from build123d import *

# Parameters (mm, degrees)
F0_W      = 6
F0_H      = 2
F1_DEPTH  = 6
F2_W      = 6
F2_H      = 6
F3_DEPTH  = 10
F4_W      = 24
F4_H      = 12
F5_DEPTH  = 6
F7_DEPTH  = 12.001
F8_W      = 6.1598163333
F8_H      = 6
F9_DEPTH  = 15
F10_W     = 6
F10_H     = 2.5150536597
F11_DEPTH = 4
F12_W     = 24.6021291241
F12_H     = 7.3056968898
F13_DEPTH = 6
F14_W     = 5.5018218607
F14_H     = 5.5230222642
F15_DEPTH = 24.6031291241
F16_R     = 1.5
F17_DEPTH = 1
F18_W     = 2.4501711503
F18_H     = 3.5
F18_W_2   = 2.5247114152
F18_W_3   = 2.5247123465
F19_DEPTH = 5


with BuildPart() as f1:
    # F0 (on Top) → F1 (new body)
    with BuildSketch(Plane.XY):
        with Locations((-32.0476180848, -1)):
            Rectangle(F0_W, F0_H)
    extrude(amount=F1_DEPTH)

    # F2 (on face) → F3 (join)
    with BuildSketch(Plane.YZ.offset(-29.0476180848)):
        with Locations((-1.0433437443, 3)):
            Rectangle(F2_W, F2_H)
    extrude(amount=F3_DEPTH)

    # F4 (on face) → F5 (join)
    with BuildSketch(Plane.YZ.offset(-19.0476180848)):
        with Locations((-1.0433437443, 3)):
            Rectangle(F4_W, F4_H)
    extrude(amount=F5_DEPTH)

    # F6 (on face) → F7 (cut, through all)
    with BuildSketch(Plane.XY.offset(9)):
        with BuildLine():
            Line((-13.0476180848, -11.1071496376), (-13.0476180848, -7.6019221608))
            ThreePointArc((-13.0476180848, -7.6019221608), (-16.5476180848, -9.3545358992), (-13.0476180848, -11.1071496376))
        make_face()
        with BuildLine():
            ThreePointArc((-13.0476180848, 0.4656811595), (-16.5476180848, -1.0765416363), (-13.0476180848, -2.618764432))
            Line((-13.0476180848, -2.618764432), (-13.0476180848, 0.4656811595))
        make_face()
        with BuildLine():
            ThreePointArc((-13.0476180848, 9.0525666852), (-16.5476180848, 7.234418936), (-13.0476180848, 5.4162711868))
            Line((-13.0476180848, 5.4162711868), (-13.0476180848, 9.0525666852))
        make_face()
    extrude(amount=-F7_DEPTH, mode=Mode.SUBTRACT)

    # F8 (on face) → F9 (join)
    with BuildSketch(Plane.XY.offset(6)):
        with Locations((-25.9677099181, -1.0433437443)):
            Rectangle(F8_W, F8_H)
    extrude(amount=F9_DEPTH)

    # F10 (on face) → F11 (join)
    with BuildSketch(Plane.YZ.offset(-22.8878017515)):
        with Locations((-1.0433437443, 19.7424731702)):
            Rectangle(F10_W, F10_H)
    extrude(amount=F11_DEPTH)

    # F12 (on face) → F13 (join)
    with BuildSketch(Plane.YZ.offset(-18.8878017515)):
        with Locations((-0.8769654669, 17.3471515551)):
            Rectangle(F12_W, F12_H)
    extrude(amount=F13_DEPTH)

    # F14 (on face) → F15 (cut, through all)
    with BuildSketch(Plane(origin=(0, 11.4240990952, 0), x_dir=(-1, 0, 0), z_dir=(0, 1, 0))):
        with Locations((15.6387126818, 17.3303969204)):
            Rectangle(F14_W, F14_H)
    extrude(amount=-F15_DEPTH, mode=Mode.SUBTRACT)

    # F16 (on face) → F17 (cut)
    with BuildSketch(Plane.XY.offset(14.5688857883)):
        with Locations((-13.8878017515, -9.5042175321)):
            Circle(F16_R)
        with Locations((-13.8878017515, -1.0522056698)):
            Circle(F16_R)
        with Locations((-13.8878017515, 7.322568293)):
            Circle(F16_R)
    extrude(amount=-F17_DEPTH, mode=Mode.SUBTRACT)

    # F18 (on face) → F19 (join)
    with BuildSketch(Plane(origin=(0, 0, 20.0919080526), x_dir=(1, 0, 0), z_dir=(0, 0, -1))):
        with Locations((-14.1128873266, -7.338691324)):
            Rectangle(F18_W, F18_H)
        with Locations((-14.1501574591, 1.0843175156)):
            Rectangle(F18_W_2, F18_H)
        with Locations((-14.1501579247, 9.5073256567)):
            Rectangle(F18_W_3, F18_H)
    extrude(amount=F19_DEPTH)


solid = f1.part
The listing builds one solid part. Answer for the finished solid, in the listing's coordinates (mm). A direction names the side the tool comes from. Round coordinates to 2 decimals unless told otherwise and drop trailing zeros. Write each loop counter-clockwise with the first axis right and the second up, starting at its lowest first coordinate (ties: lowest second). Pieces come first, ordered by that corner, then holes. Notation, with made-up numbers: (-26.5, 77.25) - (27.5, 77.25) arc R25 ccw to (27.5, 104.25) - close; hole circle Ø8 at (54.5, 40). An arc over 180 degrees is marked (long way). Use a Markdown table: item, result. Add a question column.
1. The part is cut by section A-A (y = -6.75). Write down the section's boundary in (x, z), and give its area (3 significant figures).
2. Consider line 1 (Y direction, x = -14.5, z = 6.5); line 2 (Z direction, x = -16, y = 2.5); line 3 (X direction, y = 1, z = 15.5). Determine where each line is inside the solid, lowest interval first.
3. A tool of negligible diameter and unlimited length cuts with its end or side. For faces 5 (the face through (-15.413, -9, 18)), 6 (the face through (-15.387, 7.371, 14.138)), 7 (the face through (-32, -1, 6)), from which of +Z, -Z, +X, -X, +Y, -Y can it reach the whole face along a straight path? Write none if from no direction.
4. The part is cut by section B-B (z = 5.5). Write down the section's boundary in (x, y), and give its area (3 significant figures).
5. The part is cut by section D-D (x = -28.5). Write down the section's boundary in (y, z).
6. For a pull along Z with two mould halves and no side action, classify faces 1 (the face through (-21, -1, 6)), 2 (the face through (-25, -1, 0)), 3 (the face through (-12.888, 10, 14)), 4 (the face through (-19, -1, 21)) as +Z half, -Z half, draft (parallel to the pull), parting line (faces both ways), or undercut.
7. The part is cut by section C-C (x = -15.75). Write down the section's boundary in (y, z).
8. Flat-ended cylindrical pins translate along their axes: P1, Ø5, axis at y = 0, z = 10, coming from the -X side; P2, Ø2, axis at x = -14.5, y = -2, coming from the -Z side; P3, Ø2, axis at x = -32.5, y = -1, coming from the +Z side; P4, Ø12, axis at y = 3, z = 4.5, coming from the -X side. Find the tip coordinate at first contact, or state that the pin passes through.
Reported:
| question | item | result |
|---|---|---|
| 1 | outline | (-19.05, -3) - (-13.05, -3) - (-13.05, 9) - (-19.05, 9) - close; (-18.89, 13.69) - (-12.89, 13.69) - (-12.89, 14.57) - (-18.39, 14.57) - (-18.39, 20.09) - (-12.89, 20.09) - (-12.89, 21) - (-18.89, 21) - close |
| 1 | area | 85.4 mm^2 |
| 2 | line 1 | -13.04 to -11.54, -7.17 to -3.17, 1.01 to 5.02, 9.45 to 10.96 |
| 2 | line 2 | -3 to 9, 13.69 to 14.57, 20.09 to 21 |
| 2 | line 3 | -29.05 to -22.89, -18.89 to -18.39 |
| 3 | face 5 | +Y, -Y |
| 3 | face 6 | -Z |
| 3 | face 7 | +Z, -X, +Y, -Y |
| 4 | outline | (-35.05, -2) - (-29.05, -2) - (-29.05, -4.04) - (-19.05, -4.04) - (-19.05, -13.04) - (-13.05, -13.04) - (-13.05, -11.11) arc R2.19 cw (long way) to (-13.05, -7.6) - (-13.05, -2.62) arc R2.09 cw (long way) to (-13.05, 0.47) - (-13.05, 5.42) arc R2.22 cw (long way) to (-13.05, 9.05) - (-13.05, 10.96) - (-19.05, 10.96) - (-19.05, 1.96) - (-29.05, 1.96) - (-29.05, 0) - (-35.05, 0) - close |
| 4 | area | 178 mm^2 |
| 5 | outline | (-4.04, 0) - (1.96, 0) - (1.96, 21) - (-4.04, 21) - close |
| 6 | face 1 | undercut |
| 6 | face 2 | -Z half |
| 6 | face 3 | draft |
| 6 | face 4 | +Z half |
| 7 | outline | (-13.18, 13.69) - (11.42, 13.69) - (11.42, 14.57) - (-13.18, 14.57) - close; (-13.18, 20.09) - (11.42, 20.09) - (11.42, 21) - (-13.18, 21) - close; (-13.04, -3) - (-11.04, -3) - (-11.04, 9) - (-13.04, 9) - close; (-7.66, -3) - (-2.72, -3) - (-2.72, 9) - (-7.66, 9) - close; (0.57, -3) - (5.53, -3) - (5.53, 9) - (0.57, 9) - close; (8.94, -3) - (10.96, -3) - (10.96, 9) - (8.94, 9) - close |
| 8 | P1 | x = -29.05 |
| 8 | P2 | z = 13.69 |
| 8 | P3 | z = 6 |
| 8 | P4 | x = -35.05 |
